Check sheet for the modelled part. Datum: model origin and axes. Units: mm. A direction names the side the tool comes from. Round coordinates to 2 decimals unless told otherwise and drop trailing zeros. Loops run counter-clockwise (first coordinate to the right, second up) from the corner with the lowest first, then second, coordinate; pieces in that order, holes last. Notation, with made-up numbers: (71.5, 29) - (86.5, 29) arc R24 cw to (86.5, 40) - close; hole circle Ø1 at (-29.75, 74.25). An arc over 180 degrees is marked (long way). Put each result on its own line as item: value.
```python
from build123d import *

# Parameters (mm, degrees)
F1_DEPTH = 5
F2_R     = 1.5
F3_DEPTH = 18.5
F4_R     = 3
F5_DEPTH = 3


with BuildPart() as f1:
    # F0 (on Top) → F1 (new body)
    with BuildSketch(Plane.XY):
        with BuildLine():
            ThreePointArc((0, 4.5), (3.181981, 3.181981), (4.5, 0))
            ThreePointArc((4.5, 0), (3.181981, -3.181981), (0, -4.5))
            Line((0, -4.5), (6, -4.5))
            Line((6, -4.5), (6, 4.5))
            Line((6, 4.5), (0, 4.5))
        make_face()
        with BuildLine():
            ThreePointArc((0, -4.5), (3.181981, -3.181981), (4.5, 0))
            ThreePointArc((4.5, 0), (3.181981, 3.181981), (0, 4.5))
            ThreePointArc((0, 4.5), (-4.5, 0), (0, -4.5))
        make_face()
    extrude(amount=F1_DEPTH)

    # F2 (on Top) → F3 (cut)
    with BuildSketch(Plane.XY):
        Circle(F2_R)
    extrude(amount=F3_DEPTH, mode=Mode.SUBTRACT)

    # F4 (on Top) → F5 (cut)
    with BuildSketch(Plane.XY):
        Circle(F4_R)
    extrude(amount=F5_DEPTH, mode=Mode.SUBTRACT)


solid = f1.part
```
Item 1: Go/stop test with flat-tipped pins: pin 1 (1.5 mm diameter, centred on y = 3, z = 2.5, fed in from -X); pin 2 (3 mm diameter, centred on x = 1, y = -1, fed in from -Z). Record where each tip stops, or that it passes through.
Filled sheet:
pin 1: x = -3.9
pin 2: z = 3
Item 2: Tool access check on faces 1 (the cylindrical face through (-3, 0, 1)), 2 (the flat face through (3, 1, 0)). Record the directions out of +Z, -Z, +X, -X, +Y, -Y that give a thin tool (end or side, any length) a straight path to the whole face; none if there is none.
Filled sheet:
face 1: -Z
face 2: -Z, +X, -X, +Y, -Y
Item 3: Section check D-D on y = 1.75. Enter the section's corners in (x, z).
Filled sheet:
outline: (-4.15, 0) - (-2.44, 0) - (-2.44, 3) - (2.44, 3) - (2.44, 0) - (6, 0) - (6, 5) - (-4.15, 5) - close
Item 4: Thickness scan on line 1 (X direction, y = 0, z = 3.95); line 2 (Y direction, x = 0, z = 4.6); line 3 (Y direction, x = 0, z = 1.6). Record the ranges inside material, lowest first. Write a range as from..to.
Filled sheet:
line 1: -4.5..-1.5, 1.5..6
line 2: -4.5..-1.5, 1.5..4.5
line 3: -4.5..-3, 3..4.5
Item 5: Release check for a two-part mould opening along X. For faces 3 (the flat face through (6, 0, 2)), 4 (the cylindrical face through (-4.5, 0.1, 2.5)), 5 (the flat face through (1.3, -1.3, 3)), 6 (the flat face through (2, 0, 5)) record: +X half, -X half, draft (parallel to the pull), parting line (faces both ways), or undercut.
Filled sheet:
face 3: +X half
face 4: -X half
face 5: undercut
face 6: draft
Item 6: Section check C-C on z = 0.8. Enter the section's corners in (x, y).
Filled sheet:
outline: (0, -4.5) - (6, -4.5) - (6, 4.5) - (0, 4.5) arc R4.5 ccw to start; hole circle Ø6 at (0, 0)
Item 7: Section check A-A on y = 0. Enter the section's corners in (x, z), then the cut area to 3 significant figures.
Filled sheet:
outline: (-4.5, 0) - (-3, 0) - (-3, 3) - (-1.5, 3) - (-1.5, 5) - (-4.5, 5) - close; (1.5, 3) - (3, 3) - (3, 0) - (6, 0) - (6, 5) - (1.5, 5) - close
area: 28.5 mm²
Item 8: Section check B-B on x = 1.25. Enter the section's corners in (y, z), then the cut area to 3 significant figures.
Filled sheet:
outline: (-4.5, 0) - (-2.73, 0) - (-2.73, 3) - (-0.83, 3) - (-0.83, 5) - (-4.5, 5) - close; (0.83, 3) - (2.73, 3) - (2.73, 0) - (4.5, 0) - (4.5, 5) - (0.83, 5) - close
area: 25.3 mm²
